```python
from build123d import *

# Parameters (mm, degrees)
SKETCH1_R           = 1.65
BOSS_EXTRUDE1_DEPTH = 3
SKETCH3_W           = 20
SKETCH3_H           = 3.526384588
BOSS_EXTRUDE2_DEPTH = 3


with BuildPart() as part:
    # Sketch1 → Boss-Extrude1 (new body)
    with BuildSketch(Plane.XY):
        with BuildLine():
            ThreePointArc((60, 6.136005382), (64.924934056, 0), (60, -6.136005382))
            add(Edge.make_bspline(
                [(0, -10), (30.892479525, -13.337059616), (60, -6.136005382)],
                knots=[0, 0, 0, 0.860506177, 0.860506177, 0.860506177], degree=2))
            ThreePointArc((0, -10), (7.982090261, 0), (0, 10))
            add(Edge.make_bspline(
                [(0, 10), (30.892479525, 13.337059616), (60, 6.136005382)],
                knots=[0, 0, 0, 0.860506177, 0.860506177, 0.860506177], degree=2))
        make_face()
        with Locations((12, 0)):
            Circle(SKETCH1_R, mode=Mode.SUBTRACT)
        with Locations((16, 0)):
            Circle(SKETCH1_R, mode=Mode.SUBTRACT)
        with Locations((20, 0)):
            Circle(SKETCH1_R, mode=Mode.SUBTRACT)
        with Locations((24, 0)):
            Circle(SKETCH1_R, mode=Mode.SUBTRACT)
        with Locations((54, 0)):
            Circle(SKETCH1_R, mode=Mode.SUBTRACT)
    extrude(amount=BOSS_EXTRUDE1_DEPTH)

    # Sketch3 → Boss-Extrude2 (add)
    with BuildSketch(Plane(origin=(0, 0, 0), x_dir=(-1, 0, 0), z_dir=(0, 0, -1))):
        with Locations((-39.233748341, 0)):
            Rectangle(SKETCH3_W, SKETCH3_H)
    extrude(amount=BOSS_EXTRUDE2_DEPTH)


solid = part.part
```
Geometry: final body of the model. Coordinates: model frame, mm. A direction names the side the tool comes from. Round coordinates to 2 decimals unless told otherwise and drop trailing zeros. Loops run counter-clockwise (first coordinate to the right, second up) from the corner with the lowest first, then second, coordinate; pieces in that order, holes last. Notation, with made-up numbers: (86.25, 60.5) -> (144.25, 60.5) arc R27 ccw to (144.25, 83.5) -> close; hole circle Ø10 at (89, 57). An arc over 180 degrees is marked (long way). Use one line per item in the form item = value. Start each with the question number.
1) First-contact query: P1, Ø1.5, axis at x = 32, y = 3.5, coming from the -Z side; P2, Ø4, axis at x = 20, y = 0, coming from the +Z side; P3, Ø3.5, axis at y = 0, z = -2, coming from the -X side; P4, Ø1, axis at y = 1, z = 0.5, coming from the -X side. Flat tips, straight axial feed; report the tip coordinate or a pass-through.
2) Section C-C on z = -1.75. Output: boundary loops of the cut face in (x, y).
3) Section A-A on y = 0. Output: boundary loops of the cut face in (x, z), then the cut area to 3 significant figures.
4) Access query for faces 5 (the flat face through (33, 0, 3)), 6 (the flat face through (39, 1.763, -1)). Directions: +Z, -Z, +X, -X, +Y, -Y. A direction counts if a zero-diameter tool reaches every point of the face in a straight line with its end or side. Return the directions, or none.
5) Draft query along X for faces 1 (the flat face through (49.234, 0, -1)), 2 (the cylindrical face through (52.35, 0.07, 1.48)), 3 (the flat face through (39, -1.763, -1)), 4 (the flat face through (29.234, 0, -1)). Return one class per face: released by +X, released by -X, zero draft, split by the parting line, or undercut.
6) Section D-D on y = 5.5. Output: boundary loops of the cut face in (x, z), then the cut area to 3 significant figures.
7) Section B-B on z = 1. Give the number of separate pieces and of enclosed holes in the cut face, then the cut area to 3 significant figures.
8) Line query: L1, parallel to Z at x = 47, y = 2.5; L2, parallel to Y at x = 17.5, z = 0.75; L3, parallel to Y at x = 18, z = 2.25. Output: solid intervals per line, ascending.
Response:
q1.P1 = 0
q1.P2 = 3
q1.P3 = 29.23
q1.P4 = 7.87
q2.outline = (29.23, -1.76) -> (49.23, -1.76) -> (49.23, 1.76) -> (29.23, 1.76) -> close
q3.outline = (7.98, 0) -> (10.35, 0) -> (10.35, 3) -> (7.98, 3) -> close; (13.65, 0) -> (14.35, 0) -> (14.35, 3) -> (13.65, 3) -> close; (17.65, 0) -> (18.35, 0) -> (18.35, 3) -> (17.65, 3) -> close; (21.65, 0) -> (22.35, 0) -> (22.35, 3) -> (21.65, 3) -> close; (25.65, 0) -> (29.23, 0) -> (29.23, -3) -> (49.23, -3) -> (49.23, 0) -> (52.35, 0) -> (52.35, 3) -> (25.65, 3) -> close; (55.65, 0) -> (64.92, 0) -> (64.92, 3) -> (55.65, 3) -> close
q3.area = 181 mm^2
q4.face_5 = +Z, +X, -X, +Y, -Y
q4.face_6 = -Z, +X, -X, +Y
q5.face_1 = released by +X
q5.face_2 = undercut
q5.face_3 = zero draft
q5.face_4 = released by -X
q6.outline = (6.38, 0) -> (61.68, 0) -> (61.68, 3) -> (6.38, 3) -> close
q6.area = 166 mm^2
q7.separate_pieces = 1
q7.enclosed_holes = 5
q7.area = 1,060 mm^2
q8.L1 = 0 to 3
q8.L2 = -11.05 to -0.69, 0.69 to 11.05
q8.L3 = -11.05 to 11.05
